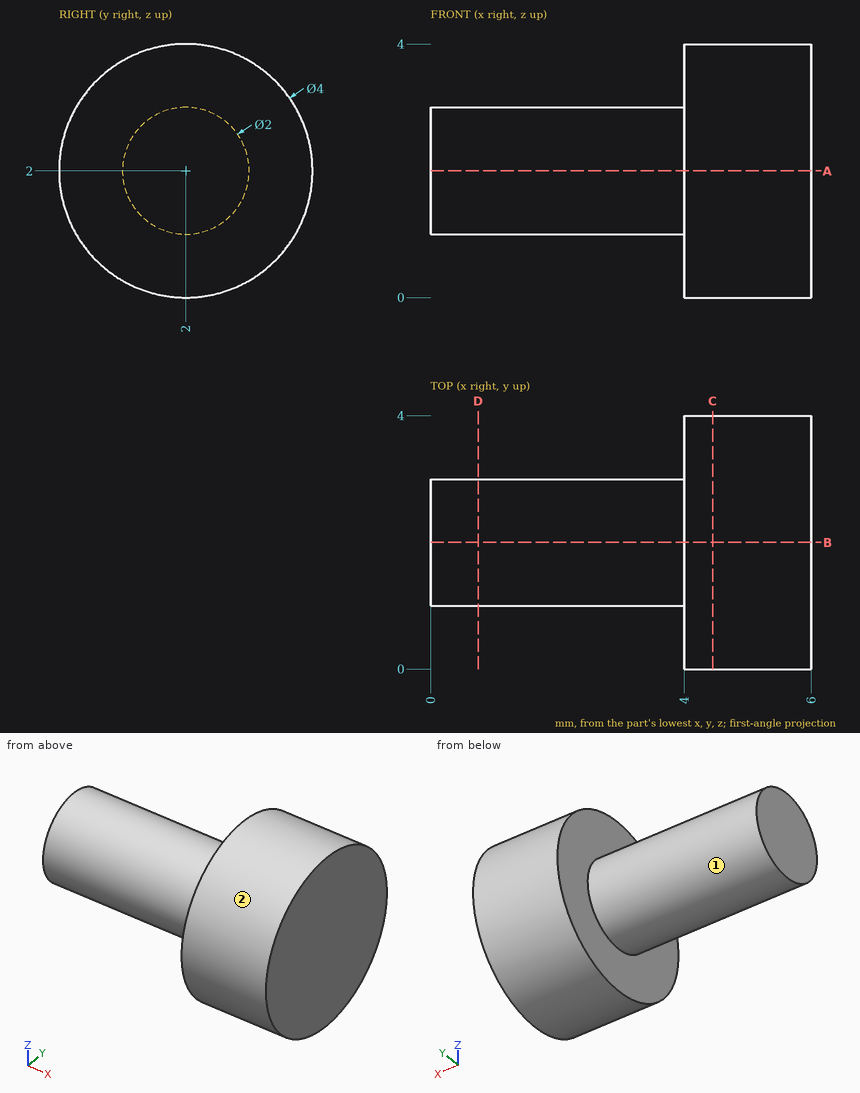
Design review of the part shown in the three views and the two pictorial views. Dimensions are in mm from the part's minimum x, y and z. A direction names the side the tool comes from. Round coordinates to 2 decimals unless told otherwise and drop trailing zeros. Write each loop counter-clockwise with the first axis right and the second up, starting at its lowest first coordinate (ties: lowest second). Pieces come first, ordered by that corner, then holes. Notation, with made-up numbers: (46, 7.25) - (55, 7.25) arc R15 cw to (55, 12.25) - close; hole circle Ø7 at (80.5, 41.25). An arc over 180 degrees is marked (long way). Write item = value, one per line. Start each with the question number.
1. Consider section C-C on x = 4.45. State the section outline as (y, z) points.
2. Consider section D-D on x = 0.75. State the section outline as (y, z) points, plus the area to 3 significant figures.
3. For the marked faces 1 and 2, list the 3-axis set-ups (+Z, -Z, +X, -X, +Y, -Y) from which the entire face can be reached by the end or side of a thin tool; tool diameter is ignored.
4. For pin 1 Ø1 at (x, z) = (1.5, 2) entering from -Y; pin 2 Ø1.5 at (x, z) = (3.5, 0.5) entering from -Y, all flat-tipped, find the tip position at first contact; note any pin that passes through.
5. Consider section A-A on z = 2. State the section outline as (x, y) points, plus the area to 3 significant figures.
6. Wall thickness on L1, parallel to X at y = 0.75, z = 2.8; L2, parallel to Y at x = 3.25, z = 1.95; L3, parallel to Z at x = 4.7, y = 0.55: over which ranges is each line inside the solid? List them lowest first.
Evaluation:
q1.outline = circle Ø4 at (2, 2)
q2.outline = circle Ø2 at (2, 2)
q2.area = 3.14 mm2
q3.face_1 = -X
q3.face_2 = +X, -X
q4.pin_1 = 1
q4.pin_2 = 0.24
q5.outline = (0, 1) - (4, 1) - (4, 0) - (6, 0) - (6, 4) - (4, 4) - (4, 3) - (0, 3) - close
q5.area = 16.0 mm2
q6.L1 = 4 to 6
q6.L2 = 1 to 3
q6.L3 = 0.62 to 3.38
